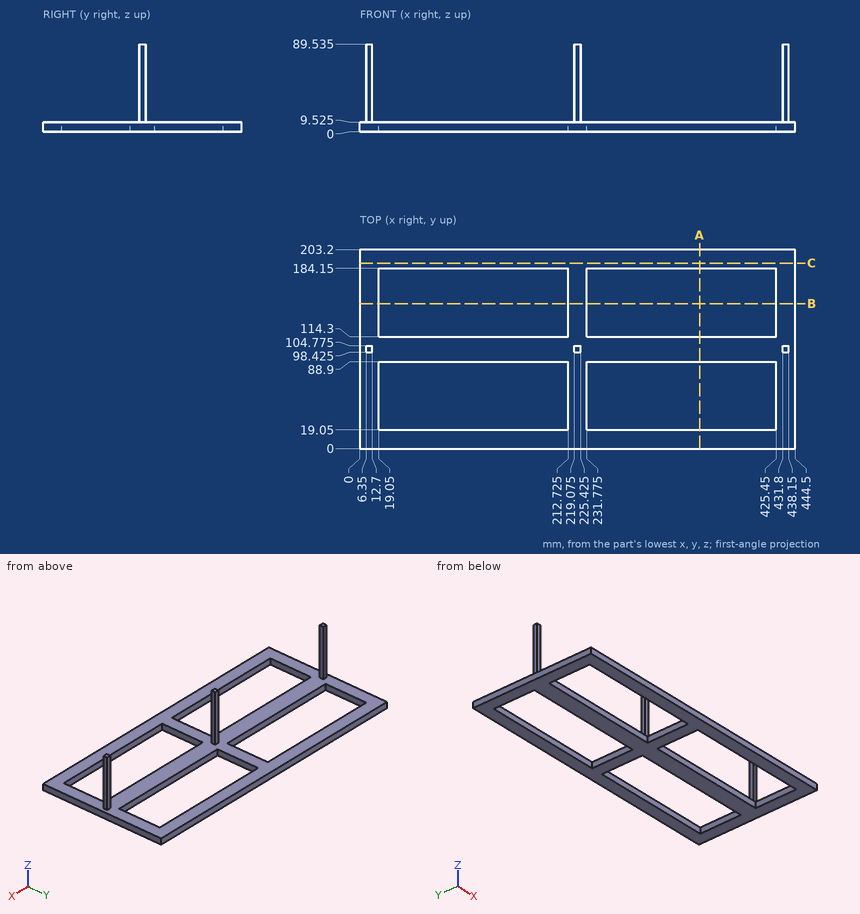
Job drawing, mm, ordinate dimensions from the low corner. One solid piece. Round coordinates to 2 decimals unless told otherwise and drop trailing zeros. Write each loop counter-clockwise with the first axis right and the second up, starting at its lowest first coordinate (ties: lowest second). Pieces come first, ordered by that corner, then holes.
1) Band-saw the part on C-C, the plane y = 189.5. List the corners of the cut face in (x, z) (3 decimals).
2) Pin check, flat tips, straight feed: pin 1 (5 mm diameter, centred on y = 103, z = 39.5, fed in from +X); pin 2 (5 mm diameter, centred on y = 100.5, z = 66, fed in from -X); pin 3 (3 mm diameter, centred on x = 9.5, z = 57.5, fed in from +Y) (3 decimals). Stop position of each tip, or through.
3) Band-saw the part on B-B, the plane y = 148. List the corners of the cut face in (x, z) (3 decimals).
4) Band-saw the part on A-A, the plane x = 347. List the corners of the cut face in (y, z) (3 decimals).
5) Drill centre lines: probe 1 along X at (y, z) = (99.5, 31.5) (3 decimals); probe 2 along Z at (x, y) = (200, 113.5) (3 decimals); probe 3 along Y at (x, z) = (223, 33.5) (3 decimals). Where is each one in solid material? Low to high.
Ans:
1. outline: (0, 0) - (444.5, 0) - (444.5, 9.525) - (0, 9.525) - close
2. pin 1: stops at x = 438.15
2. pin 2: stops at x = 6.35
2. pin 3: stops at y = 104.775
3. outline: (0, 0) - (19.05, 0) - (19.05, 9.525) - (0, 9.525) - close; (212.725, 0) - (231.775, 0) - (231.775, 9.525) - (212.725, 9.525) - close; (425.45, 0) - (444.5, 0) - (444.5, 9.525) - (425.45, 9.525) - close
4. outline: (0, 0) - (19.05, 0) - (19.05, 9.525) - (0, 9.525) - close; (88.9, 0) - (114.3, 0) - (114.3, 9.525) - (88.9, 9.525) - close; (184.15, 0) - (203.2, 0) - (203.2, 9.525) - (184.15, 9.525) - close
5. probe 1: x = 6.35 to 12.7, 219.075 to 225.425, 431.8 to 438.15
5. probe 2: z = 0 to 9.525
5. probe 3: y = 98.425 to 104.775
